Input: part model. Units: mm. Frame: model coordinates. A direction names the side the tool comes from. Coordinates: 2 decimals unless noted, no trailing zeros. Order: outer loops, then holes, each group sorted by start corner. A loop starts at its lowest first (then second) coordinate and runs counter-clockwise, first axis right, second up. Notation, with made-up numbers: M 36.25,21 L 75.25,21 A23 ccw 75.25,34 Z; hole C 10,13.5 d1. An arc over 180 degrees is marked long. Answer in a Markdown table with one row per item.
from build123d import *

# Parameters (mm, degrees)
SKETCH1_R           = 0.9
SKETCH1_R_2         = 0.65
BOSS_EXTRUDE1_DEPTH = 4
SKETCH2_W           = 16.2
SKETCH2_H           = 15.23
CUT_EXTRUDE1_DEPTH  = 2


with BuildPart() as part:
    # Sketch1 → Boss-Extrude1 (new body)
    with BuildSketch(Plane.XY):
        with BuildLine():
            Line((2, 0), (14.2, 0))
            ThreePointArc((14.2, 0), (15.614213562, 0.585786438), (16.2, 2))
            Line((16.2, 2), (16.2, 4))
            Line((16.2, 4), (12.2, 4))
            Line((12.2, 4), (12.2, 6))
            Line((12.2, 6), (16.2, 6))
            Line((16.2, 6), (16.2, 20.23))
            ThreePointArc((16.2, 20.23), (14.735533906, 23.765533906), (11.2, 25.23))
            Line((11.2, 25.23), (5, 25.23))
            ThreePointArc((5, 25.23), (1.464466094, 23.765533906), (0, 20.23))
            Line((0, 20.23), (0, 6))
            Line((0, 6), (4, 6))
            Line((4, 6), (4, 4))
            Line((4, 4), (0, 4))
            Line((0, 4), (0, 2))
            ThreePointArc((0, 2), (0.585786438, 0.585786438), (2, 0))
        make_face()
        with Locations((13.45, 2)):
            Circle(SKETCH1_R, mode=Mode.SUBTRACT)
        with Locations((13.2, 22.23)):
            Circle(SKETCH1_R_2, mode=Mode.SUBTRACT)
        with Locations((2.75, 8)):
            Circle(SKETCH1_R, mode=Mode.SUBTRACT)
        with Locations((13.45, 8)):
            Circle(SKETCH1_R, mode=Mode.SUBTRACT)
        with Locations((3, 22.23)):
            Circle(SKETCH1_R_2, mode=Mode.SUBTRACT)
        with Locations((2.75, 2)):
            Circle(SKETCH1_R, mode=Mode.SUBTRACT)
    extrude(amount=BOSS_EXTRUDE1_DEPTH)

    # Sketch2 → Cut-Extrude1 (cut)
    with BuildSketch(Plane.XY):
        with Locations((8.1, 7.615)):
            Rectangle(SKETCH2_W, SKETCH2_H)
    extrude(amount=CUT_EXTRUDE1_DEPTH, mode=Mode.SUBTRACT)


solid = part.part
1) Reachability of faces 4 (the face through (0.57, 0.6, 2.99)), 5 (the face through (2, 4, 3)), 6 (the face through (14, 4, 3)) from +Z, -Z, +X, -X, +Y, -Y: full face, straight path, thin tool, end or side. Return the list, or none.
Resolved:
| item | result |
|---|---|
| face 4 | +Z, -Z, -X, -Y |
| face 5 | +Z, -Z, -X |
| face 6 | +Z, -Z, +X |
2) Cut plane A-A, the plane z = 3.3. Output: boundary loops of the cut face in (x, y).
Resolved:
| item | result |
|---|---|
| outline | M 0,2 A2 ccw 2,0 L 14.2,0 A2 ccw 16.2,2 L 16.2,4 L 12.2,4 L 12.2,6 L 16.2,6 L 16.2,20.23 A5 ccw 11.2,25.23 L 5,25.23 A5 ccw 0,20.23 L 0,6 L 4,6 L 4,4 L 0,4 Z; hole C 2.75,2 d1.8; hole C 2.75,8 d1.8; hole C 3,22.23 d1.3; hole C 13.45,2 d1.8; hole C 13.45,8 d1.8; hole C 13.2,22.23 d1.3 |
3) Mould query, pull axis Y, two halves, no side actions, for faces 1 (the face through (8, 15.23, 1)), 2 (the face through (16.2, 14.6, 2.4)), 3 (the face through (3.6, 2.3, 3)). Classes: +Y half, -Y half, draft (parallel to the pull), parting line (faces both ways), or undercut.
Resolved:
| item | result |
|---|---|
| face 1 | -Y half |
| face 2 | draft |
| face 3 | undercut |
4) Cut plane D-D, the plane z = 1. Output: boundary loops of the cut face in (x, y).
Resolved:
| item | result |
|---|---|
| outline | M 0,15.23 L 16.2,15.23 L 16.2,20.23 A5 ccw 11.2,25.23 L 5,25.23 A5 ccw 0,20.23 Z; hole C 3,22.23 d1.3; hole C 13.2,22.23 d1.3 |
5) Cut plane B-B, the plane x = 2.75. Output: boundary loops of the cut face in (y, z), and give its area (3 significant figures).
Resolved:
| item | result |
|---|---|
| outline | M 0,2 L 1.1,2 L 1.1,4 L 0,4 Z; M 2.9,2 L 4,2 L 4,4 L 2.9,4 Z; M 6,2 L 7.1,2 L 7.1,4 L 6,4 Z; M 8.9,2 L 15.23,2 L 15.23,0 L 21.63,0 L 21.63,4 L 8.9,4 Z; M 22.83,0 L 24.7,0 L 24.7,4 L 22.83,4 Z |
| area | 52.3 mm2 |
6) Material intervals for probe 1 along X at (y, z) = (2, 2.7); probe 2 along Y at (x, z) = (3, 2.9); probe 3 along Y at (x, z) = (2.75, 3.25), sorted ascending.
Resolved:
| item | result |
|---|---|
| probe 1 | x = 0 to 1.85, 3.65 to 12.55, 14.35 to 16.2 |
| probe 2 | y = 0 to 1.14, 2.86 to 4, 6 to 7.14, 8.86 to 21.58, 22.88 to 24.81 |
| probe 3 | y = 0 to 1.1, 2.9 to 4, 6 to 7.1, 8.9 to 21.63, 22.83 to 24.7 |
7) Contact query for flat-ended pins moving along their axis: pin 1 (1 mm diameter, centred on x = 14, z = 3.5, fed in from +Y); pin 2 (1.6 mm diameter, centred on x = 14.5, z = 3.5, fed in from -Y); pin 3 (1 mm diameter, centred on x = 1.5, z = 2.5, fed in from +Y); pin 4 (2 mm diameter, centred on x = 2.75, y = 2, fed in from -Z). Output: stop coordinate, or through.
Resolved:
| item | result |
|---|---|
| pin 1 | stops at y = 24.67 |
| pin 2 | stops at y = 0 |
| pin 3 | stops at y = 24.23 |
| pin 4 | stops at z = 2 |
8) Cut plane C-C, the plane y = 22.23. Output: boundary loops of the cut face in (x, z), and give its area (3 significant figures).
Resolved:
| item | result |
|---|---|
| outline | M 0.42,0 L 2.35,0 L 2.35,4 L 0.42,4 Z; M 3.65,0 L 12.55,0 L 12.55,4 L 3.65,4 Z; M 13.85,0 L 15.78,0 L 15.78,4 L 13.85,4 Z |
| area | 51.1 mm2 |
